Could you check a few things on this model? Use its own coordinates, in mm. Coordinates: 2 decimals unless noted, no trailing zeros. Loops run counter-clockwise (first coordinate to the right, second up) from the corner with the lowest first, then second, coordinate; pieces in that order, holes last. Notation, with made-up numbers: (27.25, 86.5) -> (76.25, 86.5) arc R17 cw to (76.25, 106.5) -> close; hole circle Ø2 at (70, 39.25). An arc over 180 degrees is marked (long way). One line per question, with ' | ' between items. Start each with the question number.
(1) I'm going to push flat-ended pins straight in: pin 1 Ø1 at (y, z) = (8, 2) entering from -X; pin 2 Ø1.8 at (x, y) = (12, 0) entering from -Z. Where does each tip first touch, or does it pass through?
(2) Suppose I cut it at C-C (z = 1.5). Please give me the cut outline in (x, y).
(3) If I drill on line 1 along Y through (x, z) = (12, 1.55); line 2 along Y through (x, z) = (22, 3.85); line 3 along X through (y, z) = (4.25, 2.45), over which ranges is the centre line in solid material (lowest first)?
(4) Suppose I cut it at A-A (x = 12). Please give me the cut outline in (y, z), plus the area to 3 significant figures.
(5) Suppose I cut it at B-B (y = 0). Please give me the cut outline in (x, z), plus the area to 3 significant figures.
(6) If we mould it in two halves opening along X, with no side actions, what happens to faces 1 (the face through (0, 0, 0)), 2 (the face through (13.5, -0.07, 2.53)), 3 (the face through (-24.65, -11.49, 1.97))? For each: pulls with the +X half, pulls with the -X half, needs draft (parallel to the pull), parting line crosses it, or undercut.
```python
from build123d import *

# Parameters (mm, degrees)
F1_DEPTH = 5
F2_R     = 1
F3_D     = 3
F4_D     = 3


with BuildPart() as f1:
    # F0 (on Top) → F1 (new body)
    with BuildSketch(Plane.XY):
        with BuildLine():
            Line((17.5, 14.5), (-17.5, 14.5))
            ThreePointArc((-17.5, 14.5), (-24.5710678119, 11.5710678119), (-27.5, 4.5))
            Line((-27.5, 4.5), (-27.5, -4.5))
            ThreePointArc((-27.5, -4.5), (-24.5710678119, -11.5710678119), (-17.5, -14.5))
            Line((-17.5, -14.5), (17.5, -14.5))
            ThreePointArc((17.5, -14.5), (24.5710678119, -11.5710678119), (27.5, -4.5))
            Line((27.5, -4.5), (27.5, 4.5))
            ThreePointArc((27.5, 4.5), (24.5710678119, 11.5710678119), (17.5, 14.5))
        make_face()
    extrude(amount=F1_DEPTH)

    # F2
    f2_edges = [f1.edges().sort_by_distance(p)[0] for p in [
        (0, 14.5, 5),
        (-24.571068, 11.571068, 5),
        (-27.5, 0, 5),
        (-24.571068, -11.571068, 5),
        (0, -14.5, 5),
        (24.571068, -11.571068, 5),
        (27.5, 0, 5),
        (24.571068, 11.571068, 5),
    ]]
    fillet(f2_edges, radius=F2_R)

    # F3 (through all)
    with Locations(Plane(origin=(0, 0, 0), x_dir=(1, 0, 0), z_dir=(0, 0, -1))):
        with Locations((-21.5, -3), (21.5, -3)):
            Hole(F3_D / 2)

    # F4 (through all)
    with Locations(Plane(origin=(0, 0, 0), x_dir=(1, 0, 0), z_dir=(0, 0, -1))):
        with Locations((-12, 0), (12, 0)):
            Hole(F4_D / 2)


solid = f1.part
```
Checks:
1) pin 1: stops at x = -27.04 | pin 2: passes through
2) outline: (-27.5, -4.5) arc R10 ccw to (-17.5, -14.5) -> (17.5, -14.5) arc R10 ccw to (27.5, -4.5) -> (27.5, 4.5) arc R10 ccw to (17.5, 14.5) -> (-17.5, 14.5) arc R10 ccw to (-27.5, 4.5) -> close; hole circle Ø3 at (-21.5, 3); hole circle Ø3 at (-12, 0); hole circle Ø3 at (12, 0); hole circle Ø3 at (21.5, 3)
3) line 1: y = -14.5 to -1.5, 1.5 to 14.5 | line 2: y = -13.43 to 1.59, 4.41 to 13.43 | line 3: x = -27.5 to -22.33, -20.67 to 20.67, 22.33 to 27.5
4) outline: (-14.5, 0) -> (-1.5, 0) -> (-1.5, 5) -> (-13.5, 5) arc R1 ccw to (-14.5, 4) -> close; (1.5, 0) -> (14.5, 0) -> (14.5, 4) arc R1 ccw to (13.5, 5) -> (1.5, 5) -> close | area: 130 mm^2
5) outline: (-27.5, 0) -> (-13.5, 0) -> (-13.5, 5) -> (-26.5, 5) arc R1 ccw to (-27.5, 4) -> close; (-10.5, 0) -> (10.5, 0) -> (10.5, 5) -> (-10.5, 5) -> close; (13.5, 0) -> (27.5, 0) -> (27.5, 4) arc R1 ccw to (26.5, 5) -> (13.5, 5) -> close | area: 245 mm^2
6) face 1: needs draft | face 2: undercut | face 3: pulls with the -X half
